Geometry check sheet. Reference: drawing and pictorial views, mm from the part's lowest x, y, z. A direction names the side the tool comes from. Coordinates: 2 decimals unless noted, no trailing zeros. Loops run counter-clockwise (first coordinate to the right, second up) from the corner with the lowest first, then second, coordinate; pieces in that order, holes last.
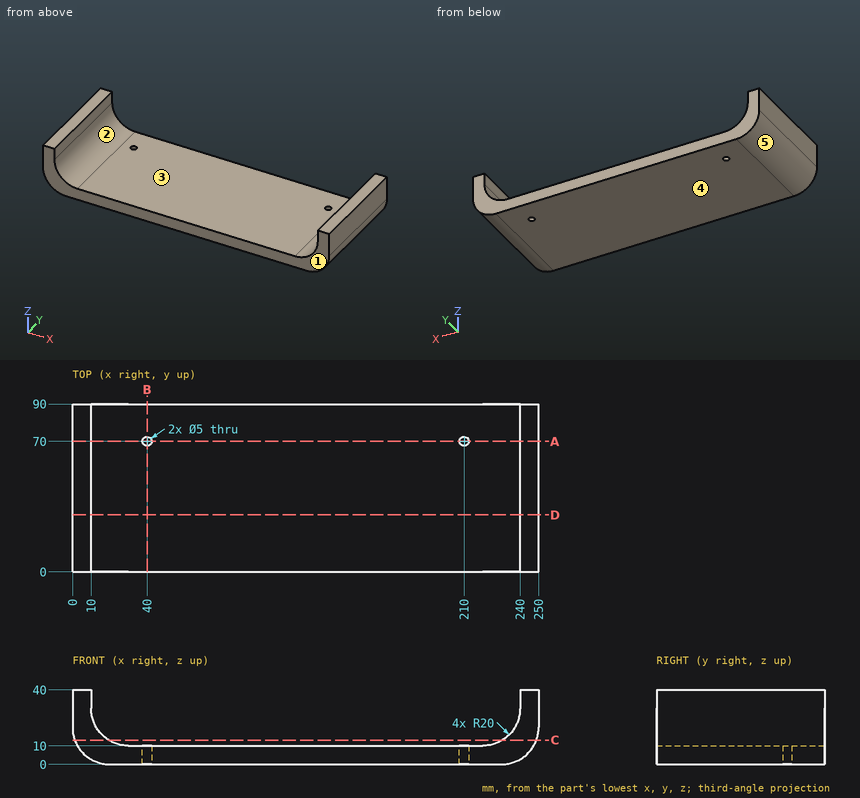
1) Material ranges on probe 1 along X at (y, z) = (56, 35.5); probe 2 along Z at (x, y) = (198, 63); probe 3 along Y at (x, z) = (40, 7.5), recorded low to high.
Data:
probe 1: x = 0 to 10, 240 to 250
probe 2: z = 0 to 10
probe 3: y = 0 to 67.5, 72.5 to 90
2) Section check A-A on y = 70. Record the cut outline in (x, z), and give its area (3 significant figures).
Data:
outline: (0, 20) arc R20 ccw to (20, 0) - (37.5, 0) - (37.5, 10) - (30, 10) arc R20 cw to (10, 30) - (10, 40) - (0, 40) - close; (42.5, 0) - (207.5, 0) - (207.5, 10) - (42.5, 10) - close; (212.5, 0) - (230, 0) arc R20 ccw to (250, 20) - (250, 40) - (240, 40) - (240, 30) arc R20 cw to (220, 10) - (212.5, 10) - close
area: 3,000 mm2
3) Access from +Z, -Z, +X, -X, +Y, -Y to the whole of each face (thin tool, end or side, straight path). Record for the marked faces 1 and 2.
Data:
face 1: +Z, -Z, +X, -X, -Y
face 2: +Z, +Y, -Y
4) Mould release check, pull along X, two halves, no side actions. Record for the marked faces 3, 4 and 5: +X half, -X half, draft (parallel to the pull), parting line (faces both ways), or undercut.
Data:
face 3: undercut
face 4: draft
face 5: -X half
5) Section check D-D on y = 30.5. Record the cut outline in (x, z), and give its area (3 significant figures).
Data:
outline: (0, 20) arc R20 ccw to (20, 0) - (230, 0) arc R20 ccw to (250, 20) - (250, 40) - (240, 40) - (240, 30) arc R20 cw to (220, 10) - (30, 10) arc R20 cw to (10, 30) - (10, 40) - (0, 40) - close
area: 3,100 mm2
6) Section check C-C on z = 13. Record the cut outline in (x, y) (3 decimals), and give its area (3 significant figures).
Data:
outline: (1.265, 0) - (19.464, 0) - (19.464, 90) - (1.265, 90) - close; (230.536, 0) - (248.735, 0) - (248.735, 90) - (230.536, 90) - close
area: 3,280 mm2
7) Section check B-B on x = 40. Record the cut outline in (y, z).
Data:
outline: (0, 0) - (67.5, 0) - (67.5, 10) - (0, 10) - close; (72.5, 0) - (90, 0) - (90, 10) - (72.5, 10) - close
8) Depth check by flat-ended pin: pin 1 (8 mm diameter, centred on x = 87.5, y = 43.5, fed in from +Z); pin 2 (8 mm diameter, centred on y = 55, z = 36, fed in from -X); pin 3 (10 mm diameter, centred on y = 71.5, z = 13, fed in from -X). Enter the tip coordinate at first touch or a pass-through.
Data:
pin 1: stops at z = 10
pin 2: stops at x = 0
pin 3: stops at x = 0.1
